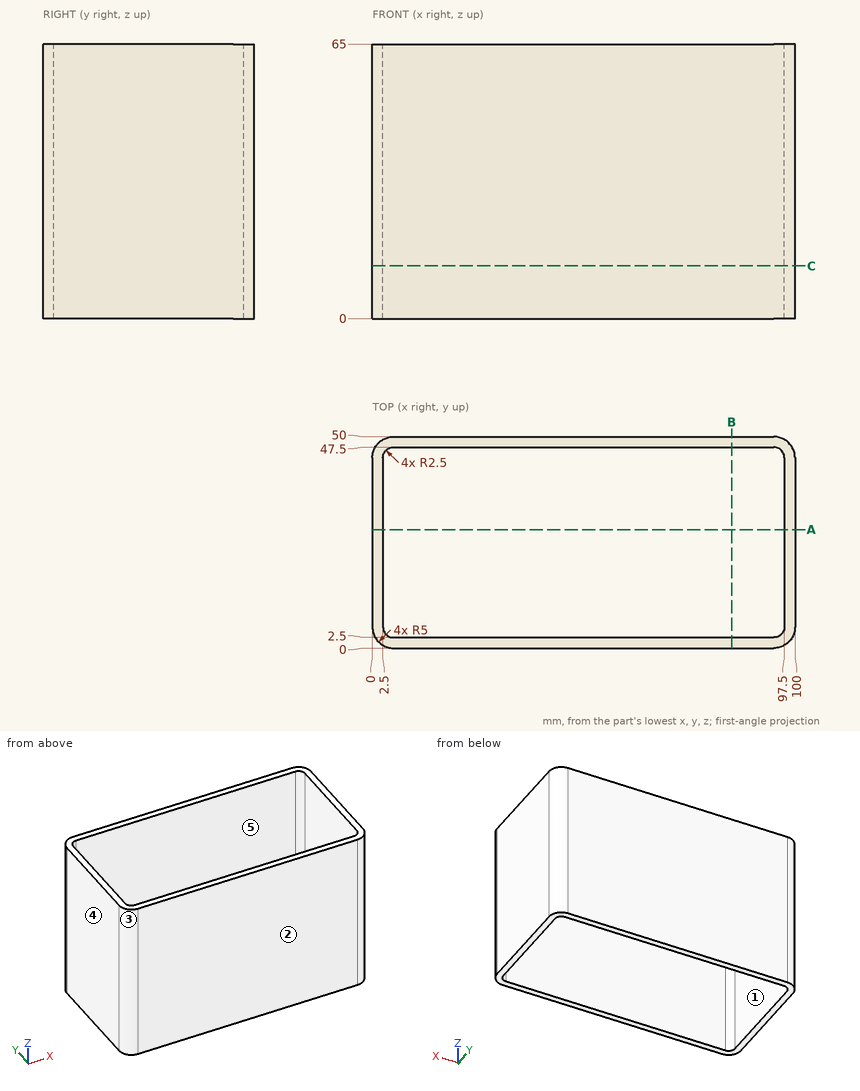
Geometry check sheet. Reference: drawing and pictorial views, mm from the part's lowest x, y, z. A direction names the side the tool comes from. Round coordinates to 2 decimals unless told otherwise and drop trailing zeros. Loops run counter-clockwise (first coordinate to the right, second up) from the corner with the lowest first, then second, coordinate; pieces in that order, holes last. Notation, with made-up numbers: (-26.75, 8.5) - (23.25, 8.5) arc R7 cw to (23.25, 15.5) - close; hole circle Ø5 at (-9.75, -30.5). An arc over 180 degrees is marked (long way). Answer as CSV lines item,"result".
(1) Set-up check for the marked faces 4 and 5: record each of +Z, -Z, +X, -X, +Y, -Y from which the full face is reachable in a straight line by a thin tool's end or side.
Output values:
face 4,"+Z, -Z, -X, +Y, -Y"
face 5,"+Z, -Z"
(2) Depth check by flat-ended pin: pin 1 Ø8 at (x, y) = (56, 8) entering from +Z. Enter the tip coordinate at first touch or a pass-through.
Output values:
pin 1,"passes through"
(3) Material ranges on line 1 along X through (y, z) = (40, 51); line 2 along Y through (x, z) = (21, 34), recorded low to high.
Output values:
line 1,"x = 0 to 2.5, 97.5 to 100"
line 2,"y = 0 to 2.5, 47.5 to 50"
(4) Release check for a two-part mould opening along X. For the marked faces 1, 2 and 3 record: released by +X, released by -X, zero draft, split by the parting line, or undercut.
Output values:
face 1,"undercut"
face 2,"zero draft"
face 3,"released by -X"
(5) Cross-section at A-A, the plane y = 28. Enter the section's corners in (x, z), and give its area (3 significant figures).
Output values:
outline,"(0, 0) - (2.5, 0) - (2.5, 65) - (0, 65) - close; (97.5, 0) - (100, 0) - (100, 65) - (97.5, 65) - close"
area,"325 mm²"
(6) Cross-section at C-C, the plane z = 12.5. Enter the section's corners in (x, y).
Output values:
outline,"(0, 5) arc R5 ccw to (5, 0) - (95, 0) arc R5 ccw to (100, 5) - (100, 45) arc R5 ccw to (95, 50) - (5, 50) arc R5 ccw to (0, 45) - close; hole (2.5, 5) arc R2.5 ccw to (5, 2.5) - (95, 2.5) arc R2.5 ccw to (97.5, 5) - (97.5, 45) arc R2.5 ccw to (95, 47.5) - (5, 47.5) arc R2.5 ccw to (2.5, 45) - close"
(7) Cross-section at B-B, the plane x = 85. Enter the section's corners in (y, z).
Output values:
outline,"(0, 0) - (2.5, 0) - (2.5, 65) - (0, 65) - close; (47.5, 0) - (50, 0) - (50, 65) - (47.5, 65) - close"
